Design review of the part built by this model. Coordinates are the model's own, in mm. Face numbers are marked on the shaded views. A direction names the side the tool comes from. Give positions to 0.01 mm unless a question says otherwise; leave off trailing zeros. Write each loop counter-clockwise with the first axis right and the second up, starting at its lowest first coordinate (ties: lowest second). Pieces come first, ordered by that corner, then holes. Notation, with made-up numbers: M 11.25,33 L 59.25,33 A22 ccw 59.25,42 Z; hole C 57.25,29 d5. An arc over 180 degrees is marked long. Write each question's results on one line, items separated by ' | '. Start each with the question number.
from build123d import *

# Parameters (mm, degrees)
CROQUIS1_W              = 110
CROQUIS1_H              = 110
CROQUIS1_W_2            = 100
CROQUIS1_H_2            = 100
SALIENTE_EXTRUIR1_DEPTH = 2
CROQUIS2_W              = 100
CROQUIS2_H              = 100
CROQUIS2_W_2            = 96
CROQUIS2_H_2            = 96
SALIENTE_EXTRUIR2_DEPTH = 4
CROQUIS3_W              = 10
CROQUIS3_H              = 96
SALIENTE_EXTRUIR3_DEPTH = 4
CROQUIS4_R              = 4
CROQUIS4_R_2            = 1
SALIENTE_EXTRUIR4_DEPTH = 20
CORTAR_EXTRUIR1_START   = -20
CROQUIS5_R              = 1
CORTAR_EXTRUIR1_DEPTH   = 20
CROQUIS6_W              = 4
CROQUIS6_H              = 2
CORTAR_EXTRUIR4_DEPTH   = 55


with BuildPart() as part:
    # Croquis1 → Saliente-Extruir1 (new body)
    with BuildSketch(Plane(origin=(0, 0, 0), x_dir=(1, 0, 0), z_dir=(0, 1, 0))):
        with Locations((50, 50)):
            Rectangle(CROQUIS1_W, CROQUIS1_H)
        with Locations((50, 50)):
            Rectangle(CROQUIS1_W_2, CROQUIS1_H_2, mode=Mode.SUBTRACT)
    extrude(amount=SALIENTE_EXTRUIR1_DEPTH)

    # Croquis2 → Saliente-Extruir2 (add)
    with BuildSketch(Plane.XZ):
        with Locations((50, -50)):
            Rectangle(CROQUIS2_W, CROQUIS2_H)
        with Locations((50, -50)):
            Rectangle(CROQUIS2_W_2, CROQUIS2_H_2, mode=Mode.SUBTRACT)
    extrude(amount=-SALIENTE_EXTRUIR2_DEPTH)

    # Croquis3 → Saliente-Extruir3 (add)
    with BuildSketch(Plane.XZ):
        with Locations((50, -50)):
            Rectangle(CROQUIS3_W, CROQUIS3_H)
    extrude(amount=-SALIENTE_EXTRUIR3_DEPTH)

    # Croquis4 → Saliente-Extruir4 (add)
    with BuildSketch(Plane(origin=(0, 4, 0), x_dir=(1, 0, 0), z_dir=(0, 1, 0))):
        with Locations(Location((50, 50, 0), (0, 0, 270))):
            Circle(CROQUIS4_R)
        with Locations(Location((50, 50, 0), (0, 0, 270))):
            Circle(CROQUIS4_R_2, mode=Mode.SUBTRACT)
    extrude(amount=SALIENTE_EXTRUIR4_DEPTH)

    # Croquis5 → Cortar-Extruir1 (cut)
    with BuildSketch(Plane(origin=(0, 4, 0), x_dir=(1, 0, 0), z_dir=(0, 1, 0)).offset(CORTAR_EXTRUIR1_START)):
        with Locations(Location((50, 50, 0), (0, 0, 270))):
            Circle(CROQUIS5_R)
    extrude(amount=CORTAR_EXTRUIR1_DEPTH, mode=Mode.SUBTRACT)

    # Croquis6 → Cortar-Extruir4 (cut)
    with BuildSketch(Plane(origin=(0, 0, -105), x_dir=(-1, 0, 0), z_dir=(0, 0, -1))):
        with Locations((-50, 1)):
            Rectangle(CROQUIS6_W, CROQUIS6_H)
    extrude(amount=-CORTAR_EXTRUIR4_DEPTH, mode=Mode.SUBTRACT)


solid = part.part
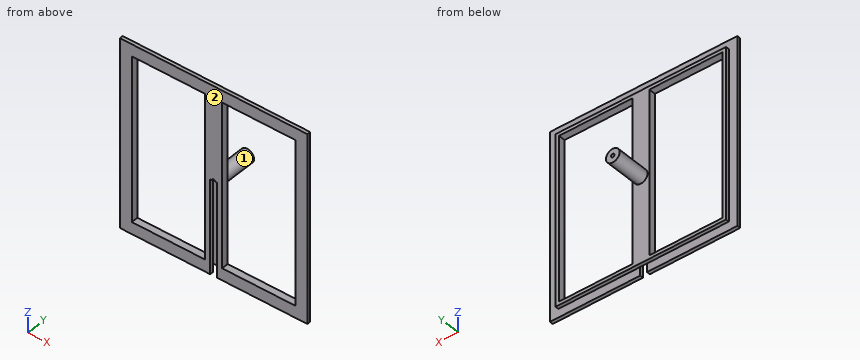
Q1. For the marked faces 1 and 2, list the 3-axis set-ups (+Z, -Z, +X, -X, +Y, -Y) from which the entire face can be reached by the end or side of a thin tool; tool diameter is ignored.
Q2. We need section C-C on z = -85. Write out the cut boundary in (x, y).
Q3. For pin 1 Ø2 at (y, z) = (2.5, -59.5) entering from +X; pin 2 Ø1.8 at (x, z) = (50, -50) entering from -Y; pin 3 Ø6 at (x, y) = (50, 13.5) entering from -Z; pin 4 Ø6 at (y, z) = (5.5, -13.5) entering from +X, all flat-tipped, find the tip position at first contact; note any pin that passes through.
Q4. Wall thickness on line 1 along X through (y, z) = (3.5, -36.5); line 2 along X through (y, z) = (13.75, -50); line 3 along Z through (x, y) = (62, 1): over which ranges is each line inside the solid? List them lowest first. Write a range as from..to.
Q5. We need section A-A on z = -41.5. Write out the cut boundary in (x, y), and give its area (3 significant figures).
Q6. We need section D-D on y = 8.25. Write out the cut boundary in (x, z), and give its area (3 significant figures).
Q7. We need section B-B on x = 29. Write out the cut boundary in (y, z).
Answer sheet:
1) face 1: +Y | face 2: +Z, -Z, +X, -X, -Y
2) outline: M -5,0 L 2,0 L 2,4 L 0,4 L 0,2 L -5,2 Z; M 45,0 L 48,0 L 48,2 L 52,2 L 52,0 L 55,0 L 55,4 L 45,4 Z; M 98,0 L 105,0 L 105,2 L 100,2 L 100,4 L 98,4 Z
3) pin 1: x = 105 | pin 2: through | pin 3: z = -54 | pin 4: x = 100
4) line 1: 0..2, 45..55, 98..100 | line 2: 46..49, 51..54 | line 3: -105..-98, -2..5
5) outline: M -5,0 L 2,0 L 2,4 L 0,4 L 0,2 L -5,2 Z; M 45,0 L 55,0 L 55,4 L 45,4 Z; M 98,0 L 105,0 L 105,2 L 100,2 L 100,4 L 98,4 Z | area: 76.0 mm^2
6) outline: C 50,-50 d8; hole C 50,-50 d2 | area: 47.1 mm^2
7) outline: M 0,-105 L 2,-105 L 2,-100 L 4,-100 L 4,-98 L 0,-98 Z; M 0,-2 L 4,-2 L 4,0 L 2,0 L 2,5 L 0,5 Z
